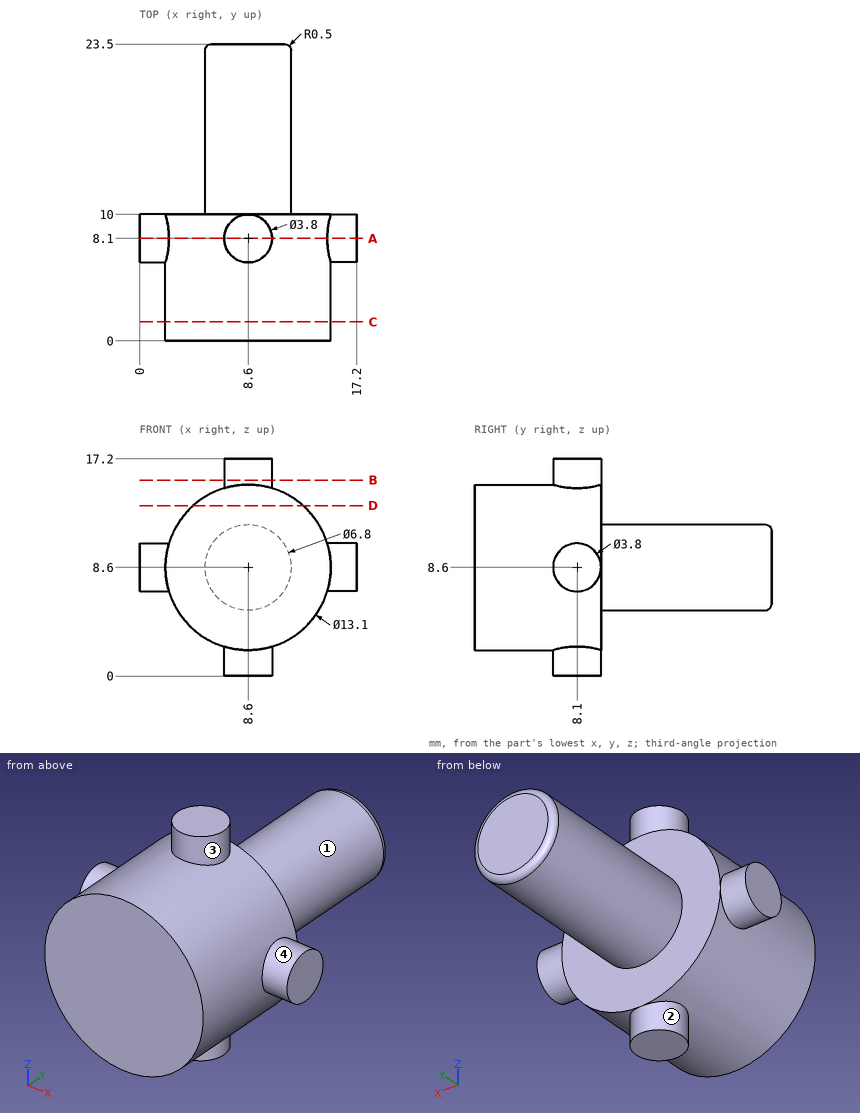
The figure shows three views and two pictorial views of one solid part (mm, origin at its lowest corner). Answer the questions. A direction names the side the tool comes from. Coordinates: 2 decimals unless noted, no trailing zeros. Write each loop counter-clockwise with the first axis right and the second up, starting at its lowest first coordinate (ties: lowest second). Pieces come first, ordered by that corner, then holes. Notation, with made-up numbers: M -5,59 L -1,59 A20 ccw -1,81 Z; hole C -7.5,50.25 d1. An arc over 180 degrees is marked long. Answer as CSV lines item,"result". Start each with the question number.
Item 1: Section D-D on z = 13.5 is taken. Write down the section's boundary in (x, y).
Item 2: Section B-B on z = 15.5 is taken. Write down the section's boundary in (x, y), and give its area (3 significant figures).
Item 3: Flat-ended cylindrical pins translate along their axes: P1, Ø10, axis at y = 15.5, z = 2, coming from the -X side; P2, Ø5, axis at y = 10.5, z = 3, coming from the -X side; P3, Ø2, axis at y = 14.5, z = 8.5, coming from the +X side. Find the tip coordinate at first contact, or state that the pin passes through.
Item 4: Section C-C on y = 1.5 is taken. Write down the section's boundary in (x, z).
Item 5: Section A-A on y = 8.1 is taken. Write down the section's boundary in (x, z), and give its area (3 significant figures).
Item 6: A tool of negligible diameter and unlimited length cuts with its end or side. For the marked faces 1, 2, 3 and 4, from which of +Z, -Z, +X, -X, +Y, -Y can it reach the whole face along a straight path? Write none if from no direction.
Item 7: Consider L1, parallel to Y at x = 8.5, z = 2.5; L2, parallel to X at y = 20.25, z = 9.5; L3, parallel to Z at x = 3.5, y = 2. Determine where each line is inside the solid, lowest interval first.
Checks:
1,outline,"M 4.25,0 L 12.95,0 L 12.95,10 L 4.25,10 Z"
2,outline,"C 8.6,8.1 d3.8"
2,area,"11.3 mm²"
3,P1,"stops at x = 5.6"
3,P2,"stops at x = 2.86"
3,P3,"stops at x = 12"
4,outline,"C 8.6,8.6 d13.1"
5,outline,"M 0,6.7 L 2.33,6.7 A6.55 ccw 6.7,2.33 L 6.7,0 L 10.5,0 L 10.5,2.33 A6.55 ccw 14.87,6.7 L 17.2,6.7 L 17.2,10.5 L 14.87,10.5 A6.55 ccw 10.5,14.87 L 10.5,17.2 L 6.7,17.2 L 6.7,14.87 A6.55 ccw 2.33,10.5 L 0,10.5 Z"
5,area,"167 mm²"
6,face 1,"+Y"
6,face 2,"-Z"
6,face 3,"+Z"
6,face 4,"+X"
7,L1,"y = 0 to 10"
7,L2,"x = 5.32 to 11.88"
7,L3,"z = 4.49 to 12.71"
